CAD build for the part. Positions are in the model's coordinates, mm. A direction names the side the tool comes from. Round coordinates to 2 decimals unless told otherwise and drop trailing zeros. Write each loop counter-clockwise with the first axis right and the second up, starting at its lowest first coordinate (ties: lowest second). Pieces come first, ordered by that corner, then holes. Notation, with made-up numbers: (78, 48.25) - (114, 48.25) arc R21 ccw to (114, 80.25) - close; hole circle Ø7 at (10.5, 26). An arc over 180 degrees is marked (long way). Put each result on its own line as item: value. Start each with the question number.
Item 1: Drill centre lines: line 1 (Z direction, x = 11.75, y = 1.75); line 2 (X direction, y = 0, z = 4); line 3 (Y direction, x = 5.5, z = 13.5). Where is each one in solid material? Low to high. Write a range as from..to.
Item 2: Cut at A-A (y = 0). Give the cut face in (x, z).
Item 3: Cut at C-C (y = 6). Give the cut face in (x, z), and give its area (3 significant figures).
Item 4: Mould opens along Z. For faces 1 (the cylindrical face through (3.77, 6.21, 14.99)), 2 (the flat face through (7, 3, 0)), 3 (the flat face through (6, 5, 14.5)) say: released by +Z, released by -Z, zero draft, split by the parting line, or undercut.
Item 5: Pin check, flat tips, straight feed: pin 1 Ø4 at (x, y) = (10, -3) entering from -Z; pin 2 Ø3 at (x, z) = (4, 11.5) entering from -Y; pin 3 Ø3 at (x, z) = (3.5, 2) entering from -Y; pin 4 Ø2 at (y, z) = (4.5, 5) entering from +X. Stop position of each tip, or through.
Item 6: Cut at D-D (x = 7.5). Give the cut face in (y, z), and give its area (3 significant figures).
Item 7: Cut at B-B (x = 4.75). Give the cut face in (y, z).
Item 8: 3-axis set-ups, long thin cutter, end or side, ignore diameter. For faces 4 (the cylindrical face through (2.5, -1.4, 10.7)), 5 (the cylindrical face through (3.77, 6.21, 3.45)): which of +Z, -Z, +X, -X, +Y, -Y reach the whole face in a straight line?
```python
from build123d import *

# Parameters (mm, degrees)
F3_DEPTH = 7.0009987
F4_DEPTH = 25.4


with BuildPart() as f1:
    # F0 (on Front) → F1 (revolve)
    with BuildSketch(Plane.XZ):
        Polygon((0, 7.0000114), (0, 0), (4.49999862, 0), (4.49999862, 15.49999948), (0, 15.49999948), (0, 14.5000218), (2.286, 14.5000218), (2.286, 7.0000114), align=None)
    revolve(axis=Axis((6.9999987, 0, 7.74999974), (0, 0, 1)))

    # F2 (on Front) → F3 (cut, through all)
    with BuildSketch(Plane.XZ):
        with BuildLine():
            Line((7.00024, 4.9995884903), (7.00024, 1.9995944903))
            ThreePointArc((7.00024, 1.9995944903), (8.0608980505, 2.4389334398), (8.500237, 3.4995914903))
            ThreePointArc((8.500237, 3.4995914903), (8.0608980505, 4.5602495407), (7.00024, 4.9995884903))
        make_face()
        with BuildLine():
            ThreePointArc((7.00024, 4.9995884903), (5.500243, 3.4995914903), (7.00024, 1.9995944903))
            Line((7.00024, 1.9995944903), (7.00024, 4.9995884903))
        make_face()
    extrude(amount=-F3_DEPTH, mode=Mode.SUBTRACT)

    # F2 (on Front) → F4 (cut)
    with BuildSketch(Plane.XZ):
        with BuildLine():
            ThreePointArc((7.00024, 4.9995884903), (5.500243, 3.4995914903), (7.00024, 1.9995944903))
            Line((7.00024, 1.9995944903), (7.00024, 4.9995884903))
        make_face()
        with BuildLine():
            Line((7.00024, 4.9995884903), (7.00024, 1.9995944903))
            ThreePointArc((7.00024, 1.9995944903), (8.0608980505, 2.4389334398), (8.500237, 3.4995914903))
            ThreePointArc((8.500237, 3.4995914903), (8.0608980505, 4.5602495407), (7.00024, 4.9995884903))
        make_face()
    extrude(amount=F4_DEPTH, mode=Mode.SUBTRACT)


solid = f1.part
```
Output values:
1. line 1: 0..7, 14.5..15.5
1. line 2: 0..4.5, 9.5..14
1. line 3: -4.47..-2, 2..4.47
2. outline: (0, 0) - (4.5, 0) - (4.5, 15.5) - (0, 15.5) - (0, 14.5) - (2.29, 14.5) - (2.29, 7) - (0, 7) - close; (9.5, 0) - (14, 0) - (14, 7) - (11.71, 7) - (11.71, 14.5) - (14, 14.5) - (14, 15.5) - (9.5, 15.5) - close
3. outline: (3.39, 0) - (10.61, 0) - (10.61, 7) - (3.39, 7) - close; (3.39, 14.5) - (10.61, 14.5) - (10.61, 15.5) - (3.39, 15.5) - close; hole circle Ø3 at (7, 3.5)
3. area: 50.6 mm2
4. face 1: zero draft
4. face 2: released by -Z
4. face 3: undercut
5. pin 1: z = 0
5. pin 2: y = -4.47
5. pin 3: y = -6.71
5. pin 4: x = 13.06
6. outline: (-6.98, 0) - (-2.45, 0) - (-2.45, 2.09) - (-6.98, 2.09) - close; (-6.98, 4.91) - (-2.45, 4.91) - (-2.45, 15.5) - (-6.98, 15.5) - (-6.98, 14.5) - (-4.69, 14.5) - (-4.69, 7) - (-6.98, 7) - close; (2.45, 0) - (6.98, 0) - (6.98, 2.09) - (2.45, 2.09) - close; (2.45, 4.91) - (6.98, 4.91) - (6.98, 7) - (4.69, 7) - (4.69, 14.5) - (6.98, 14.5) - (6.98, 15.5) - (2.45, 15.5) - close
6. area: 80.4 mm2
7. outline: (-6.63, 0) - (-1.09, 0) - (-1.09, 15.5) - (-6.63, 15.5) - (-6.63, 14.5) - (-4.14, 14.5) - (-4.14, 7) - (-6.63, 7) - close; (1.09, 0) - (6.63, 0) - (6.63, 7) - (4.14, 7) - (4.14, 14.5) - (6.63, 14.5) - (6.63, 15.5) - (1.09, 15.5) - close
8. face 4: none
8. face 5: +Z, -Z
